Could you check a few things on this model? Use its own coordinates, in mm. Give positions to 0.01 mm unless a question says otherwise; leave off trailing zeros. Loops run counter-clockwise (first coordinate to the right, second up) from the corner with the lowest first, then second, coordinate; pieces in that order, holes last. Notation, with made-up numbers: (89, 7) - (135, 7) arc R19 ccw to (135, 19) - close; hole circle Ø6 at (52.5, 59.25). An arc over 180 degrees is marked (long way). Write each question's results on one line, items separated by ' | '. Start each with the question number.
1) I want a section at B-B, the plane x = 10. Write out the boundary of the cut face in (y, z), and give its area (3 significant figures).
2) I'm going to push flat-ended pins straight in: pin 1 (0.6 mm diameter, centred on y = 10, z = -2, fed in from -X); pin 2 (0.8 mm diameter, centred on x = 8, y = 10, fed in from -Z); pin 3 (0.5 mm diameter, centred on y = 3, z = -2.5, fed in from +X). Where does each tip first touch, or does it pass through?
3) I want a section at A-A, the plane y = 7.5. Count the separate pieces of the cut face and the enclosed holes in it, and give its area (3 significant figures).
4) I want a section at C-C, the plane z = 7.5. Write out the boundary of the cut face in (x, y), and give its area (3 significant figures).
5) If I drill on probe 1 along X at (y, z) = (11, -0.25); probe 2 along Z at (x, y) = (-1.5, 11.25); probe 3 along Y at (x, z) = (-13.5, 0.25), over which ranges is the centre line in solid material (lowest first)? Write a range as [from, to].
from build123d import *

# Parameters (mm, degrees)
ESBO_O1_W                  = 32.5
ESBO_O1_H                  = 19.5
RESSALTO_EXTRUS_O1_DEPTH   = 2
RESSALTO_EXTRUS_O2_DEPTH   = 2.5
ESBO_O3_W                  = 0.75
ESBO_O3_H                  = 0.75
RESSALTO_EXTRUS_O3_DEPTH   = 9
PADR_O_LINEAR1_COUNT       = 4
PADR_O_LINEAR1_PITCH       = 2.2
PADR_O_START               = 2
PADR_O_LINEAR2_DEPTH       = 2.5
PADR_O_START_2             = 4.5
PADR_O_LINEAR2_2_OUTLINE_W = 0.75
PADR_O_LINEAR2_2_OUTLINE_H = 0.75
PADR_O_LINEAR2_2_DEPTH     = 9


# Read off the part's stored shape, not the designer's step: Padrão linear2
with BuildPart() as part:
    # Esboço1 → Ressalto-extrusão1 (new body)
    with BuildSketch(Plane(origin=(0, 0, 0), x_dir=(1, 0, 0), z_dir=(0, 1, 0))):
        Rectangle(ESBO_O1_W, ESBO_O1_H)
    extrude(amount=RESSALTO_EXTRUS_O1_DEPTH)

    # Esboço2 → Ressalto-extrusão2 (add)
    with BuildSketch(Plane(origin=(0, 2, 0), x_dir=(1, 0, 0), z_dir=(0, 1, 0))):
        Polygon((-12.851070796, 5.211508821), (-12.595390899, 5.461508821), (-10.895517077, 5.461508821), (-10.651070796, 5.211508821), (-10.651070796, 3.505955102), (-10.901070796, 3.261508821), (-12.601070796, 3.261508821), (-12.851070796, 3.517188718), align=None)
    ressalto_extrus_o2 = extrude(amount=RESSALTO_EXTRUS_O2_DEPTH)

    # Esboço3 → Ressalto-extrusão3 (add)
    with BuildSketch(Plane(origin=(0, 4.5, 0), x_dir=(1, 0, 0), z_dir=(0, 1, 0))):
        with Locations((-11.751070796, 4.358731961)):
            Rectangle(ESBO_O3_W, ESBO_O3_H)
    ressalto_extrus_o3 = extrude(amount=RESSALTO_EXTRUS_O3_DEPTH)

    # Padrão linear1: Ressalto-extrusão2, Ressalto-extrusão3 ×4
    with Locations(*[(0, 0, i * PADR_O_LINEAR1_PITCH) for i in range(1, PADR_O_LINEAR1_COUNT)]):
        add(ressalto_extrus_o2)
        add(ressalto_extrus_o3)

    # Padrão linear2 outline → Padrão linear2 (add)
    with BuildSketch(Plane(origin=(0, 0, 0), x_dir=(1, 0, 0), z_dir=(0, 1, 0)).offset(PADR_O_START)):
        Polygon((-0.895517077, 5.461508821), (-2.595390899, 5.461508821), (-2.851070796, 5.211508821), (-2.851070796, 3.517188718), (-2.598294638, 3.258669589), (-2.851070796, 3.011508821), (-2.851070796, 1.317188718), (-2.598294638, 1.058669589), (-2.851070796, 0.811508821), (-2.851070796, -0.882811282), (-2.598294638, -1.141330411), (-2.851070796, -1.388491179), (-2.851070796, -3.082811282), (-2.601070796, -3.338491179), (-0.901070796, -3.338491179), (-0.651070796, -3.094044898), (-0.651070796, -1.388491179), (-0.898231564, -1.13571502), (-0.651070796, -0.894044898), (-0.651070796, 0.811508821), (-0.898231564, 1.06428498), (-0.651070796, 1.305955102), (-0.651070796, 3.011508821), (-0.898231564, 3.26428498), (-0.651070796, 3.505955102), (-0.651070796, 5.211508821), align=None)
        Polygon((9.104482923, 5.461508821), (7.404609101, 5.461508821), (7.148929204, 5.211508821), (7.148929204, 3.517188718), (7.401705362, 3.258669589), (7.148929204, 3.011508821), (7.148929204, 1.317188718), (7.401705362, 1.058669589), (7.148929204, 0.811508821), (7.148929204, -0.882811282), (7.401705362, -1.141330411), (7.148929204, -1.388491179), (7.148929204, -3.082811282), (7.398929204, -3.338491179), (9.098929204, -3.338491179), (9.348929204, -3.094044898), (9.348929204, -1.388491179), (9.101768436, -1.13571502), (9.348929204, -0.894044898), (9.348929204, 0.811508821), (9.101768436, 1.06428498), (9.348929204, 1.305955102), (9.348929204, 3.011508821), (9.101768436, 3.26428498), (9.348929204, 3.505955102), (9.348929204, 5.211508821), align=None)
    extrude(amount=PADR_O_LINEAR2_DEPTH)

    # Padr_o linear2 2 outline → Padr_o linear2 2 (add)
    with BuildSketch(Plane(origin=(0, 0, 0), x_dir=(1, 0, 0), z_dir=(0, 1, 0)).offset(PADR_O_START_2)):
        with Locations((-1.751070796, 4.358731961)):
            Rectangle(PADR_O_LINEAR2_2_OUTLINE_W, PADR_O_LINEAR2_2_OUTLINE_H)
        with Locations((8.248929204, 4.358731961)):
            Rectangle(PADR_O_LINEAR2_2_OUTLINE_W, PADR_O_LINEAR2_2_OUTLINE_H)
        with Locations((-1.751070796, 2.158731961)):
            Rectangle(PADR_O_LINEAR2_2_OUTLINE_W, PADR_O_LINEAR2_2_OUTLINE_H)
        with Locations((8.248929204, 2.158731961)):
            Rectangle(PADR_O_LINEAR2_2_OUTLINE_W, PADR_O_LINEAR2_2_OUTLINE_H)
        with Locations((-1.751070796, -0.041268039)):
            Rectangle(PADR_O_LINEAR2_2_OUTLINE_W, PADR_O_LINEAR2_2_OUTLINE_H)
        with Locations((8.248929204, -0.041268039)):
            Rectangle(PADR_O_LINEAR2_2_OUTLINE_W, PADR_O_LINEAR2_2_OUTLINE_H)
        with Locations((-1.751070796, -2.241268039)):
            Rectangle(PADR_O_LINEAR2_2_OUTLINE_W, PADR_O_LINEAR2_2_OUTLINE_H)
        with Locations((8.248929204, -2.241268039)):
            Rectangle(PADR_O_LINEAR2_2_OUTLINE_W, PADR_O_LINEAR2_2_OUTLINE_H)
    extrude(amount=PADR_O_LINEAR2_2_DEPTH)


solid = part.part
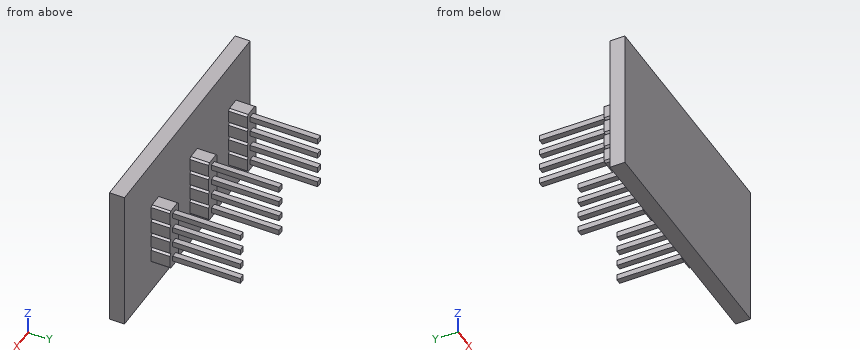
Answers:
1) outline: (0, -9.75) - (2, -9.75) - (2, 9.75) - (0, 9.75) - close | area: 39.0 mm2
2) pin 1: stops at x = -12.13 | pin 2: stops at z = -4.73 | pin 3: stops at x = 9.35
3) separate pieces: 12 | enclosed holes: 0 | area: 6.75 mm2
4) outline: (-16.25, 0) - (16.25, 0) - (16.25, 2) - (-16.25, 2) - close | area: 65.0 mm2
5) probe 1: x = [-12.13, -11.38], [-2.13, -1.38], [7.87, 8.62] | probe 2: z = [-4.73, -3.98], [-2.53, -1.78], [-0.33, 0.42], [1.87, 2.62] | probe 3: y = [0, 2]
